Print and shaded views of the part. All mm, measured from the part's lowest x, y and z. A direction names the side the tool comes from. Coordinates: 2 decimals unless noted, no trailing zeros. Order: outer loops, then holes, each group sorted by start corner. A loop starts at its lowest first (then second) coordinate and runs counter-clockwise, first axis right, second up. Notation, with made-up numbers: (-40, 58) - (-5, 58) arc R22 cw to (-5, 69) - close; hole circle Ø1 at (-30, 25). An arc over 180 degrees is marked (long way). Write each question's results on one line, items separated by ' | '.
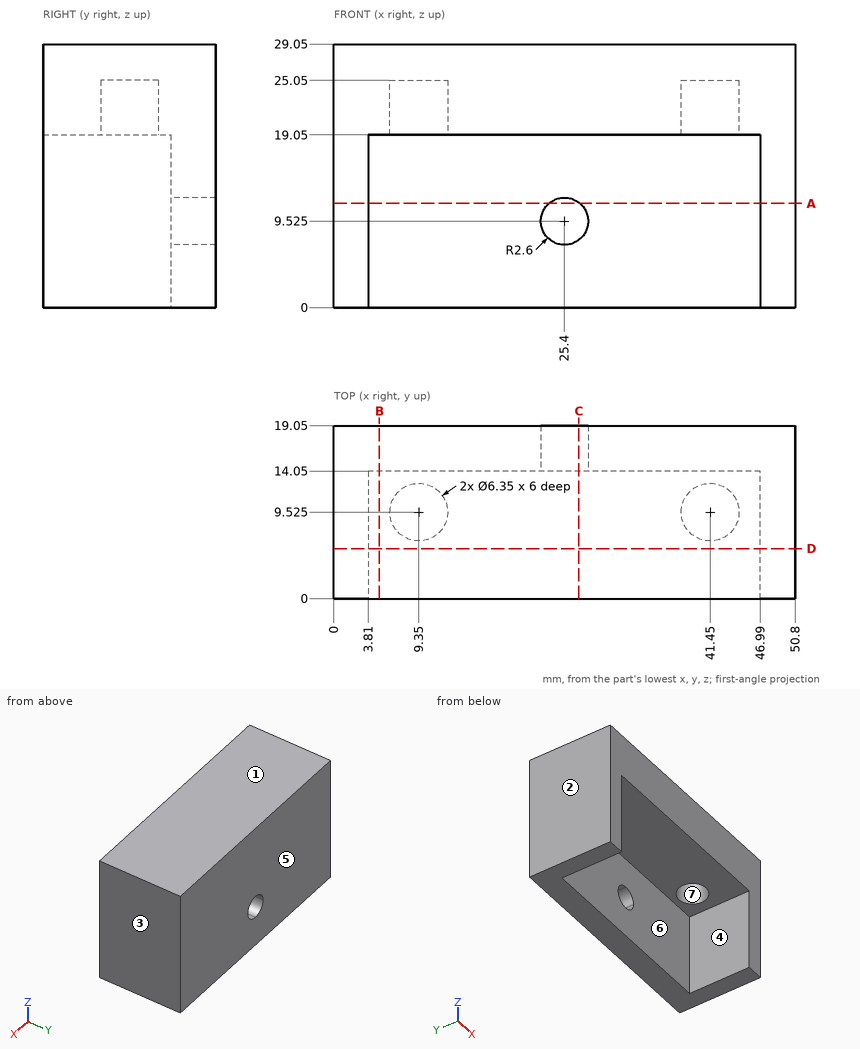
1. Tool access for the marked faces 5, 6 and 7: list every direction of +Z, -Z, +X, -X, +Y, -Y with a clear straight run to the whole face (end or side of a thin tool).
Solved:
face 5: +Z, -Z, +X, -X, +Y | face 6: -Z, -Y | face 7: -Z
2. Probe line 1 (X direction, y = 12.25, z = 8.5); line 2 (Z direction, x = 27.5, y = 1); line 3 (Y direction, x = 44, z = 25). List the from-to ranges inside material, lowest first.
Solved:
line 1: x = 0 to 3.81, 46.99 to 50.8 | line 2: z = 19.05 to 29.05 | line 3: y = 0 to 7.63, 11.42 to 19.05
3. Two-plate mould, pull along X, no slides. Class the marked faces 1, 2, 3 and 4: +X half, -X half, draft (parallel to the pull), parting line (faces both ways), or undercut.
Solved:
face 1: draft | face 2: -X half | face 3: +X half | face 4: undercut
4. Drop flat-ended pins along their axis: pin 1 Ø4 at (y, z) = (16.5, 20) entering from -X; pin 2 Ø7 at (x, y) = (10, 10) entering from -Z; pin 3 Ø3 at (x, y) = (40.5, 8.5) entering from -Z; pin 4 Ø3 at (x, z) = (39, 13.5) entering from -Y. Give the stop position or say it passes through.
Solved:
pin 1: stops at x = 0 | pin 2: stops at z = 19.05 | pin 3: stops at z = 25.05 | pin 4: stops at y = 14.05
5. Band-saw the part on D-D on y = 5.5. Give the cut face in (x, z).
Solved:
outline: (0, 0) - (3.81, 0) - (3.81, 19.05) - (46.99, 19.05) - (46.99, 0) - (50.8, 0) - (50.8, 29.05) - (0, 29.05) - close
6. Band-saw the part on B-B on x = 5. Give the cut face in (y, z).
Solved:
outline: (0, 19.05) - (14.05, 19.05) - (14.05, 0) - (19.05, 0) - (19.05, 29.05) - (0, 29.05) - close
7. Band-saw the part on C-C on x = 27. Give the cut face in (y, z), then the cut area to 3 significant figures.
Solved:
outline: (0, 19.05) - (14.05, 19.05) - (14.05, 11.57) - (19.05, 11.57) - (19.05, 29.05) - (0, 29.05) - close; (14.05, 0) - (19.05, 0) - (19.05, 7.48) - (14.05, 7.48) - close | area: 265 mm2
8. Band-saw the part on A-A on z = 11.5. Give the cut face in (x, y).
Solved:
outline: (0, 0) - (3.81, 0) - (3.81, 14.05) - (23.71, 14.05) - (23.71, 19.05) - (0, 19.05) - close; (27.09, 14.05) - (46.99, 14.05) - (46.99, 0) - (50.8, 0) - (50.8, 19.05) - (27.09, 19.05) - close
